from build123d import *

# Parameters (mm, degrees)
ESQUISSE1_R        = 2.15
BOSS_EXTRU_1_DEPTH = 456


with BuildPart() as part:
    # Esquisse1 → Boss.-Extru.1 (new, symmetric)
    with BuildSketch(Plane(origin=(0, 0, 0), x_dir=(-1, 0, 0), z_dir=(0, 0, -1))):
        with BuildLine():
            Line((-40, 6.7), (-40, 2))
            ThreePointArc((-40, 2), (-39.414213562, 0.585786438), (-38, 0))
            Line((-38, 0), (-33.3, 0))
            ThreePointArc((-33.3, 0), (-32.734314575, 0.234314575), (-32.5, 0.8))
            Line((-32.5, 0.8), (-32.5, 1.5))
            ThreePointArc((-32.5, 1.5), (-32.587867966, 1.712132034), (-32.8, 1.8))
            Line((-32.8, 1.8), (-34.918424061, 1.8))
            ThreePointArc((-34.918424061, 1.8), (-35.686700051, 2.313345604), (-35.506437047, 3.219588924))
            Line((-35.506437047, 3.219588924), (-33.254705627, 5.471320344))
            ThreePointArc((-33.254705627, 5.471320344), (-32.281435581, 6.121638598), (-31.133385284, 6.35))
            Line((-31.133385284, 6.35), (-28.866614716, 6.35))
            ThreePointArc((-28.866614716, 6.35), (-27.718564419, 6.121638598), (-26.745294373, 5.471320344))
            Line((-26.745294373, 5.471320344), (-24.493562953, 3.219588924))
            ThreePointArc((-24.493562953, 3.219588924), (-24.313299949, 2.313345604), (-25.081575939, 1.8))
            Line((-25.081575939, 1.8), (-27.2, 1.8))
            ThreePointArc((-27.2, 1.8), (-27.412132034, 1.712132034), (-27.5, 1.5))
            Line((-27.5, 1.5), (-27.5, 0.8))
            ThreePointArc((-27.5, 0.8), (-27.265685425, 0.234314575), (-26.7, 0))
            Line((-26.7, 0), (-13.3, 0))
            ThreePointArc((-13.3, 0), (-12.734314575, 0.234314575), (-12.5, 0.8))
            Line((-12.5, 0.8), (-12.5, 1.5))
            ThreePointArc((-12.5, 1.5), (-12.587867966, 1.712132034), (-12.8, 1.8))
            Line((-12.8, 1.8), (-14.918424061, 1.8))
            ThreePointArc((-14.918424061, 1.8), (-15.686700051, 2.313345604), (-15.506437047, 3.219588924))
            Line((-15.506437047, 3.219588924), (-13.254705627, 5.471320344))
            ThreePointArc((-13.254705627, 5.471320344), (-12.281435581, 6.121638598), (-11.133385284, 6.35))
            Line((-11.133385284, 6.35), (-8.866614716, 6.35))
            ThreePointArc((-8.866614716, 6.35), (-7.718564419, 6.121638598), (-6.745294373, 5.471320344))
            Line((-6.745294373, 5.471320344), (-4.493562953, 3.219588924))
            ThreePointArc((-4.493562953, 3.219588924), (-4.313299949, 2.313345604), (-5.081575939, 1.8))
            Line((-5.081575939, 1.8), (-7.2, 1.8))
            ThreePointArc((-7.2, 1.8), (-7.412132034, 1.712132034), (-7.5, 1.5))
            Line((-7.5, 1.5), (-7.5, 0.8))
            ThreePointArc((-7.5, 0.8), (-7.265685425, 0.234314575), (-6.7, 0))
            Line((-6.7, 0), (-2, 0))
            ThreePointArc((-2, 0), (-0.585786438, 0.585786438), (0, 2))
            Line((0, 2), (0, 6.7))
            ThreePointArc((0, 6.7), (-0.234314575, 7.265685425), (-0.8, 7.5))
            Line((-0.8, 7.5), (-1.5, 7.5))
            ThreePointArc((-1.5, 7.5), (-1.712132034, 7.412132034), (-1.8, 7.2))
            Line((-1.8, 7.2), (-1.8, 5.081575939))
            ThreePointArc((-1.8, 5.081575939), (-2.313345604, 4.313299949), (-3.219588924, 4.493562953))
            Line((-3.219588924, 4.493562953), (-5.471320344, 6.745294373))
            ThreePointArc((-5.471320344, 6.745294373), (-6.121638598, 7.718564419), (-6.35, 8.866614716))
            Line((-6.35, 8.866614716), (-6.35, 11.133385284))
            ThreePointArc((-6.35, 11.133385284), (-6.121638598, 12.281435581), (-5.471320344, 13.254705627))
            Line((-5.471320344, 13.254705627), (-3.219588924, 15.506437047))
            ThreePointArc((-3.219588924, 15.506437047), (-2.313345604, 15.686700051), (-1.8, 14.918424061))
            Line((-1.8, 14.918424061), (-1.8, 12.8))
            ThreePointArc((-1.8, 12.8), (-1.712132034, 12.587867966), (-1.5, 12.5))
            Line((-1.5, 12.5), (-0.8, 12.5))
            ThreePointArc((-0.8, 12.5), (-0.234314575, 12.734314575), (0, 13.3))
            Line((0, 13.3), (0, 18))
            ThreePointArc((0, 18), (-0.585786438, 19.414213562), (-2, 20))
            Line((-2, 20), (-6.7, 20))
            ThreePointArc((-6.7, 20), (-7.265685425, 19.765685425), (-7.5, 19.2))
            Line((-7.5, 19.2), (-7.5, 18.5))
            ThreePointArc((-7.5, 18.5), (-7.412132034, 18.287867966), (-7.2, 18.2))
            Line((-7.2, 18.2), (-5.081575939, 18.2))
            ThreePointArc((-5.081575939, 18.2), (-4.313299949, 17.686654396), (-4.493562953, 16.780411076))
            Line((-4.493562953, 16.780411076), (-6.745294373, 14.528679656))
            ThreePointArc((-6.745294373, 14.528679656), (-7.718564419, 13.878361402), (-8.866614716, 13.65))
            Line((-8.866614716, 13.65), (-11.133385284, 13.65))
            ThreePointArc((-11.133385284, 13.65), (-12.281435581, 13.878361402), (-13.254705627, 14.528679656))
            Line((-13.254705627, 14.528679656), (-15.506437047, 16.780411076))
            ThreePointArc((-15.506437047, 16.780411076), (-15.686700051, 17.686654396), (-14.918424061, 18.2))
            Line((-14.918424061, 18.2), (-12.8, 18.2))
            ThreePointArc((-12.8, 18.2), (-12.587867966, 18.287867966), (-12.5, 18.5))
            Line((-12.5, 18.5), (-12.5, 19.2))
            ThreePointArc((-12.5, 19.2), (-12.734314575, 19.765685425), (-13.3, 20))
            Line((-13.3, 20), (-26.7, 20))
            ThreePointArc((-26.7, 20), (-27.265685425, 19.765685425), (-27.5, 19.2))
            Line((-27.5, 19.2), (-27.5, 18.5))
            ThreePointArc((-27.5, 18.5), (-27.412132034, 18.287867966), (-27.2, 18.2))
            Line((-27.2, 18.2), (-25.081575939, 18.2))
            ThreePointArc((-25.081575939, 18.2), (-24.313299949, 17.686654396), (-24.493562953, 16.780411076))
            Line((-24.493562953, 16.780411076), (-26.745294373, 14.528679656))
            ThreePointArc((-26.745294373, 14.528679656), (-27.718564419, 13.878361402), (-28.866614716, 13.65))
            Line((-28.866614716, 13.65), (-31.133385284, 13.65))
            ThreePointArc((-31.133385284, 13.65), (-32.281435581, 13.878361402), (-33.254705627, 14.528679656))
            Line((-33.254705627, 14.528679656), (-35.506437047, 16.780411076))
            ThreePointArc((-35.506437047, 16.780411076), (-35.686700051, 17.686654396), (-34.918424061, 18.2))
            Line((-34.918424061, 18.2), (-32.8, 18.2))
            ThreePointArc((-32.8, 18.2), (-32.587867966, 18.287867966), (-32.5, 18.5))
            Line((-32.5, 18.5), (-32.5, 19.2))
            ThreePointArc((-32.5, 19.2), (-32.734314575, 19.765685425), (-33.3, 20))
            Line((-33.3, 20), (-38, 20))
            ThreePointArc((-38, 20), (-39.414213562, 19.414213562), (-40, 18))
            Line((-40, 18), (-40, 13.3))
            ThreePointArc((-40, 13.3), (-39.765685425, 12.734314575), (-39.2, 12.5))
            Line((-39.2, 12.5), (-38.5, 12.5))
            ThreePointArc((-38.5, 12.5), (-38.287867966, 12.587867966), (-38.2, 12.8))
            Line((-38.2, 12.8), (-38.2, 14.918424061))
            ThreePointArc((-38.2, 14.918424061), (-37.686654396, 15.686700051), (-36.780411076, 15.506437047))
            Line((-36.780411076, 15.506437047), (-34.528679656, 13.254705627))
            ThreePointArc((-34.528679656, 13.254705627), (-33.878361402, 12.281435581), (-33.65, 11.133385284))
            Line((-33.65, 11.133385284), (-33.65, 8.866614716))
            ThreePointArc((-33.65, 8.866614716), (-33.878361402, 7.718564419), (-34.528679656, 6.745294373))
            Line((-34.528679656, 6.745294373), (-36.780411076, 4.493562953))
            ThreePointArc((-36.780411076, 4.493562953), (-37.686654396, 4.313299949), (-38.2, 5.081575939))
            Line((-38.2, 5.081575939), (-38.2, 7.2))
            ThreePointArc((-38.2, 7.2), (-38.287867966, 7.412132034), (-38.5, 7.5))
            Line((-38.5, 7.5), (-39.2, 7.5))
            ThreePointArc((-39.2, 7.5), (-39.765685425, 7.265685425), (-40, 6.7))
        make_face()
        with Locations((-10, 10)):
            Circle(ESQUISSE1_R, mode=Mode.SUBTRACT)
        with Locations((-30, 10)):
            Circle(ESQUISSE1_R, mode=Mode.SUBTRACT)
        with BuildLine():
            Line((-18.585786174, 17.312993861), (-14.528681072, 13.255889759))
            ThreePointArc((-14.528681072, 13.255889759), (-13.878362627, 12.282619622), (-13.650001154, 11.134569154))
            Line((-13.650001154, 11.134569154), (-13.650001154, 8.865431094))
            ThreePointArc((-13.650001154, 8.865431094), (-13.878362476, 7.717381202), (-14.5286805, 6.7441115))
            Line((-14.5286805, 6.7441115), (-18.585786, 2.687006))
            ThreePointArc((-18.585786, 2.687006), (-19.999999562, 2.101219562), (-21.414213125, 2.687006))
            Line((-21.414213125, 2.687006), (-25.471320125, 6.744113))
            ThreePointArc((-25.471320125, 6.744113), (-26.121638379, 7.717383046), (-26.349999781, 8.865433344))
            Line((-26.349999781, 8.865433344), (-26.349999781, 11.134567344))
            ThreePointArc((-26.349999781, 11.134567344), (-26.121638308, 12.282617811), (-25.471319863, 13.255887949))
            Line((-25.471319863, 13.255887949), (-21.41421295, 17.312993861))
            ThreePointArc((-21.41421295, 17.312993861), (-19.999999562, 17.898780125), (-18.585786174, 17.312993861))
        make_face(mode=Mode.SUBTRACT)
    extrude(amount=BOSS_EXTRU_1_DEPTH, both=True)


solid = part.part
Can you work these out from the model? Positions are in its coordinate system, mm. Round coordinates to 2 decimals unless told otherwise and drop trailing zeros. Use a Markdown table: item, result.
Item 1: I want a section at A-A (z = -208.5). State how many separate pieces and enclosed holes the cut face has, and give its area (3 significant figures).
Found:
| item | result |
|---|---|
| separate pieces | 1 |
| enclosed holes | 3 |
| area | 332 mm2 |
Item 2: If I drill on line 1 along X through (y, z) = (9.5, 348); line 2 along X through (y, z) = (5.5, 14); line 3 along Y through (x, z) = (37.5, -400), over which ranges is the centre line in solid material (lowest first)? Write a range as [from, to].
Found:
| item | result |
|---|---|
| line 1 | x = [6.35, 7.91], [12.09, 13.65], [26.35, 27.91], [32.09, 33.65] |
| line 2 | x = [0, 1.8], [4.23, 6.77], [13.23, 15.77], [24.23, 26.77], [33.23, 35.77], [38.2, 40] |
| line 3 | y = [0, 4.26], [15.74, 20] |
Item 3: For pin 1 Ø1.8 at (y, z) = (10, -5.5) entering from +X; pin 2 Ø0.6 at (y, z) = (1, -145.5) entering from -X; pin 3 Ø2.5 at (x, z) = (10.5, 195.5) entering from +Y, each with a flat end and sliding along its axis, tell me the tip position at first contact or that it passes through.
Found:
| item | result |
|---|---|
| pin 1 | stops at x = 33.65 |
| pin 2 | stops at x = 0.13 |
| pin 3 | stops at y = 13.71 |
